Part model, mm, in its own coordinate system. Coordinates: 2 decimals unless noted, no trailing zeros. Write each loop counter-clockwise with the first axis right and the second up, starting at its lowest first coordinate (ties: lowest second). Pieces come first, ordered by that corner, then holes. Notation, with made-up numbers: (39.5, 85) -> (93.5, 85) arc R8 ccw to (93.5, 92) -> close; hole circle Ø10 at (-20.75, 79). An arc over 180 degrees is marked (long way). Write item = value, one per line.
from build123d import *

# Parameters (mm, degrees)
F1_DEPTH = 19.05
F3_D     = 5.0038
F3_DEPTH = 14.224
F3_TIP   = 1.5032931827


with BuildPart() as f1:
    # F0 (on Right) → F1 (new body)
    with BuildSketch(Plane.YZ):
        with BuildLine():
            Line((304.8, -622.3), (304.8, 622.3))
            Line((304.8, 622.3), (124.6301678728, 622.3))
            ThreePointArc((124.6301678728, 622.3), (114.5071784324, 621.2811719909), (104.7902356525, 618.2655545193))
            Line((104.7902356525, 618.2655545193), (-304.8, 444.5))
            Line((-304.8, 444.5), (-304.8, 396.875))
            Line((-304.8, 396.875), (-304.8, -622.3))
            Line((-304.8, -622.3), (304.8, -622.3))
        make_face()
    extrude(amount=F1_DEPTH)

    # F3
    with Locations(Plane.YZ.offset(19.05)):
        with Locations((-203.2, 136.525), (-203.2, 104.775), (-203.2, 73.025), (-203.2, 41.275), (-203.2, 9.525), (-203.2, -22.225), (-203.2, -53.975), (-203.2, -85.725), (-203.2, -117.475), (-203.2, -149.225), (-203.2, -180.975), (-203.2, -212.725), (-203.2, -244.475), (-203.2, -276.225), (-203.2, -307.975), (-203.2, -339.725), (-203.2, -371.475), (-203.2, -403.225), (203.2, -403.225), (203.2, -371.475), (203.2, -339.725), (203.2, -307.975), (203.2, -276.225), (203.2, -244.475), (203.2, -212.725), (203.2, -180.975), (203.2, -149.225), (203.2, -117.475), (203.2, -85.725), (203.2, -53.975), (203.2, -22.225), (203.2, 9.525), (203.2, 41.275), (203.2, 73.025), (203.2, 104.775), (203.2, 136.525)):
            Hole(F3_D / 2, depth=F3_DEPTH)
            with Locations((0, 0, -(F3_DEPTH + F3_TIP / 2))):  # 118° drill point
                Cone(0, F3_D / 2, F3_TIP, mode=Mode.SUBTRACT)


with BuildPart() as f4_1:
    # F4: instance of F1
    add(f1.part.mirror(Plane(origin=(9.525, 304.8, 0), x_dir=(-1, 0, 0), z_dir=(0, 1, 0))))


solid = f4_1.part
Q1. Saw through at A-A on y = 745.5. Give the cut face in (x, z), and give its area (3 significant figures).
Model answer:
outline = (0, -622.3) -> (19.05, -622.3) -> (19.05, 516.15) -> (0, 516.15) -> close
area = 21,700 mm²
Q2. Saw through at B-B on x = 9. Count the separate pieces of the cut face and the enclosed holes in it, and give its area (3 significant figures).
Model answer:
separate_pieces = 1
enclosed_holes = 36
area = 721,000 mm²
Q3. Saw through at C-C on z = 463. Give the cut face in (x, y), and give its area (3 significant figures).
Model answer:
outline = (0, 304.8) -> (19.05, 304.8) -> (19.05, 870.79) -> (0, 870.79) -> close
area = 10,800 mm²
Q4. Pin check, flat tips, straight feed: pin 1 (4 mm diameter, centred on y = 406.4, z = -22.225, fed in from +X); pin 2 (3 mm diameter, centred on y = 812.8, z = 104.775, fed in from +X); pin 3 (4.5 mm diameter, centred on y = 812.8, z = 41.275, fed in from +X). Stop position of each tip, or through.
Model answer:
pin_1 = 4.52
pin_2 = 4.22
pin_3 = 4.67
Q5. Probe line 1 (Z direction, x = 10.75, y = 571); line 2 (Z direction, x = 6.5, y = 875.5); line 3 (Y direction, x = 6.25, z = 473.5). List the from-to ranges inside material, lowest first. Write a range as from..to.
Model answer:
line_1 = -622.3..590.18
line_2 = -622.3..461
line_3 = 304.8..846.04
